Source: CAD feature listing. Evaluate the final solid. Frame: model axes, mm. Face numbers are marked on the shaded views. A direction names the side the tool comes from. Coordinates: 2 decimals unless noted, no trailing zeros. Write each loop counter-clockwise with the first axis right and the second up, starting at its lowest first coordinate (ties: lowest second). Pieces come first, ordered by that corner, then holes. Notation, with made-up numbers: (20.5, 60) - (27.5, 60) arc R27 ccw to (27.5, 86) - close; hole circle Ø5 at (79.25, -20.75). An arc over 180 degrees is marked (long way). One line per question, with ' | ' between items. Start each with the question number.
Q1. Cut plane B-B, the plane x = 0. Give the number of separate pieces and of enclosed holes in the cut face, plus the area to 3 significant figures.
Q2. Access query for the marked faces 1 and 2. Directions: +Z, -Z, +X, -X, +Y, -Y. A direction counts if a zero-diameter tool reaches every point of the face in a straight line with its end or side. Return the directions, or none.
Q3. Contact query for flat-ended pins moving along their axis: P1, Ø4, axis at x = -1, z = -5, coming from the +Y side; P2, Ø0.7, axis at x = 1, y = 23.5, coming from the +Z side. Output: stop coordinate, or through.
Q4. Cut plane A-A, the plane z = -6.75. Return loops of the section in (x, y).
Q5. Line query: line 1 (Y direction, x = 0, z = -5.5); line 2 (X direction, y = 20.5, z = -0.5); line 3 (Y direction, x = -0.5, z = -5). Output: solid intervals per line, ascending.
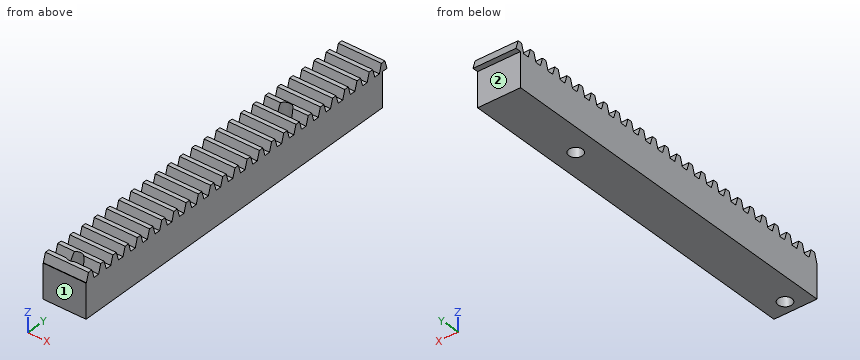
```python
from build123d import *

# Parameters (mm, degrees)
SKETCH_1_W             = 8
SKETCH_1_H             = 85
EXTRUDE_1_DEPTH        = 5
EXTRUDE_2_DEPTH        = 5
PATTERN_LINEAR_1_COUNT = 51
PATTERN_LINEAR_1_PITCH = 3.5
SKETCH_3_R             = 1.6
CUT_EXTRUDE_1_DEPTH    = 46.204424562


with BuildPart() as part:
    # 草图1 → 凸台-拉伸1 (new, symmetric)
    with BuildSketch(Plane(origin=(0, 0, 0), x_dir=(0, 0, -1), z_dir=(1, 0, 0))):
        with Locations((4, 0)):
            Rectangle(SKETCH_1_W, SKETCH_1_H)
    extrude(amount=EXTRUDE_1_DEPTH, both=True)

    # 草图2 → 凸台-拉伸2 (add, symmetric)
    with BuildSketch(Plane(origin=(0, 0, 0), x_dir=(0, 0, -1), z_dir=(1, 0, 0))):
        Polygon((0, -42.4), (-2, -41.8), (-2, -40.8), (0, -40.2), align=None)
    extrude_2 = extrude(amount=EXTRUDE_2_DEPTH, both=True)

    # 阵列(线性)1: 凸台-拉伸2 ×51, 26 skipped
    with Locations(*[(0, i * PATTERN_LINEAR_1_PITCH, 0) for i in range(1, PATTERN_LINEAR_1_COUNT) if i not in (25, 26, 27, 28, 29, 30, 31, 32, 33, 34, 35, 36, 37, 38, 39, 40, 41, 42, 43, 44, 45, 46, 47, 48, 49, 50)]):
        add(extrude_2)

    # 草图3 → 切除-拉伸1 (cut, through all)
    with BuildSketch(Plane(origin=(0, 0, -8), x_dir=(-1, 0, 0), z_dir=(0, 0, -1))):
        with Locations((0, -39.5)):
            Circle(SKETCH_3_R)
        with Locations((0, 20.5)):
            Circle(SKETCH_3_R)
        with Locations((0, 80.5)):
            Circle(SKETCH_3_R)
    extrude(amount=-CUT_EXTRUDE_1_DEPTH, mode=Mode.SUBTRACT)


solid = part.part
```
Reply:
1) separate pieces: 3 | enclosed holes: 0 | area: 704 mm^2
2) face 1: +Z, -Z, +X, -X, -Y | face 2: -Z, +X, -X, +Y
3) P1: stops at y = 42.5 | P2: stops at z = 0
4) outline: (-5, -42.5) - (5, -42.5) - (5, 42.5) - (-5, 42.5) - close; hole circle Ø3.2 at (0, -39.5); hole circle Ø3.2 at (0, 20.5)
5) line 1: y = -42.5 to -41.1, -37.9 to 18.9, 22.1 to 42.5 | line 2: x = -5 to -1.6, 1.6 to 5 | line 3: y = -42.5 to -41.02, -37.98 to 18.98, 22.02 to 42.5
